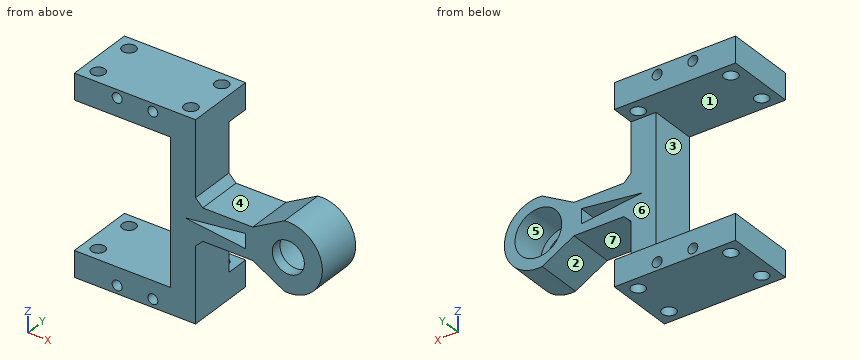
from build123d import *

# Parameters (mm, degrees)
SKETCH8_R                      = 4.5
SKETCH8_R_2                    = 1.4
BOSS_EXTRUDE2_DEPTH            = 19.5
SKETCH10_R                     = 6.55
CUT_EXTRUDE6_DEPTH             = 16.5
CUT_EXTRUDE7_DEPTH             = 43
CUT_EXTRUDE7_DEPTH_BACK        = 47
SKETCH12_R                     = 1.9
CUT_EXTRUDE8_REACH             = 79.29
SKETCH13_W                     = 46.335828735
SKETCH13_H                     = 6.5
CUT_EXTRUDE8_DIRECTION_2_REACH = 79.29
CHAMFER2_SIZE                  = 2
CUT_EXTRUDE9_DEPTH             = 13


with BuildPart() as part:
    # Sketch8 → Boss-Extrude2 (new body)
    with BuildSketch(Plane(origin=(0, 0, 0), x_dir=(1, 0, 0), z_dir=(0, 1, 0))):
        with BuildLine():
            Line((34, 4.5), (50, 4.5))
            Line((50, 4.5), (58.907986832, 9.487360394))
            ThreePointArc((58.907986832, 9.487360394), (69.55, 0), (58.907986832, -9.487360394))
            Line((58.907986832, -9.487360394), (50, -4.5))
            Line((50, -4.5), (34, -4.5))
            Line((34, -4.5), (34, -27.5))
            Line((34, -27.5), (0, -27.5))
            Line((0, -27.5), (0, -20.25))
            Line((0, -20.25), (27, -20.25))
            Line((27, -20.25), (27, 20.25))
            Line((27, 20.25), (0, 20.25))
            Line((0, 20.25), (0, 27.5))
            Line((0, 27.5), (34, 27.5))
            Line((34, 27.5), (34, 4.5))
        make_face()
        with Locations(Location((60, 0, 0), (0, 0, 270))):
            Circle(SKETCH8_R, mode=Mode.SUBTRACT)
        with Locations(Location((22, 25.25, 0), (0, 0, 270))):
            Circle(SKETCH8_R_2, mode=Mode.SUBTRACT)
        with Locations(Location((12, 25.25, 0), (0, 0, 270))):
            Circle(SKETCH8_R_2, mode=Mode.SUBTRACT)
        with Locations(Location((22, -25.25, 0), (0, 0, 270))):
            Circle(SKETCH8_R_2, mode=Mode.SUBTRACT)
        with Locations(Location((12, -25.25, 0), (0, 0, 270))):
            Circle(SKETCH8_R_2, mode=Mode.SUBTRACT)
    extrude(amount=BOSS_EXTRUDE2_DEPTH)

    # Sketch10 → Cut-Extrude6 (cut)
    with BuildSketch(Plane(origin=(0, 19.5, 0), x_dir=(1, 0, 0), z_dir=(0, 1, 0))):
        with Locations(Location((60, 0, 0), (0, 0, 270))):
            Circle(SKETCH10_R)
    extrude(amount=-CUT_EXTRUDE6_DEPTH, mode=Mode.SUBTRACT)

    # Sketch12 → Cut-Extrude7 (cut, two sides: drawn at the far end of the back side and taken through both)
    with BuildSketch(Plane.XY.offset(-CUT_EXTRUDE7_DEPTH_BACK)):
        with Locations(Location((4, 15.75, 0), (0, 0, 180))):
            Circle(SKETCH12_R)
        with Locations(Location((4, 3.75, 0), (0, 0, 180))):
            Circle(SKETCH12_R)
        with Locations(Location((30, 15.75, 0), (0, 0, 180))):
            Circle(SKETCH12_R)
        with Locations(Location((30, 3.75, 0), (0, 0, 180))):
            Circle(SKETCH12_R)
    extrude(amount=CUT_EXTRUDE7_DEPTH + CUT_EXTRUDE7_DEPTH_BACK, mode=Mode.SUBTRACT)

    # Cut-Extrude8: up to this face of the body (flat: up to its plane)
    cut_extrude8_end = Plane(part.part.faces().sort_by_distance((13.927698034, 9.75, -20.25))[0])
    # Sketch13 → Cut-Extrude8 (cut, up to the picked face)
    with BuildSketch(Plane.XY, mode=Mode.PRIVATE) as cut_extrude8_sk1:
        with Locations((46.382085633, 16.25)):
            Rectangle(SKETCH13_W, SKETCH13_H)
    cut_extrude8_tool1 = split(extrude(cut_extrude8_sk1.sketch, amount=-CUT_EXTRUDE8_REACH, mode=Mode.PRIVATE), bisect_by=cut_extrude8_end, keep=Keep.BOTH, mode=Mode.PRIVATE)
    add(cut_extrude8_tool1.solids().sort_by(Axis((46.382086, 16.25, 0), (0, 0, -1)))[0], mode=Mode.SUBTRACT)

    # Cut-Extrude8 direction 2: up to this face of the body (flat: up to its plane)
    cut_extrude8_direction_2_end = Plane(part.part.faces().sort_by_distance((13.927698034, 9.75, 20.25))[0])
    # Sketch13 → Cut-Extrude8 direction 2 (cut, up to the picked face)
    with BuildSketch(Plane.XY, mode=Mode.PRIVATE) as cut_extrude8_direction_2_sk1:
        with Locations((46.382085633, 16.25)):
            Rectangle(SKETCH13_W, SKETCH13_H)
    cut_extrude8_direction_2_tool1 = split(extrude(cut_extrude8_direction_2_sk1.sketch, amount=CUT_EXTRUDE8_DIRECTION_2_REACH, mode=Mode.PRIVATE), bisect_by=cut_extrude8_direction_2_end, keep=Keep.BOTH, mode=Mode.PRIVATE)
    add(cut_extrude8_direction_2_tool1.solids().sort_by(Axis((46.382086, 16.25, 0), (0, 0, 1)))[0], mode=Mode.SUBTRACT)

    # Chamfer2
    chamfer2_edges = [part.edges().sort_by_distance(p)[0] for p in [
        (34, 6.5, 4.5),
        (34, 6.5, -4.5),
    ]]
    chamfer(chamfer2_edges, length=CHAMFER2_SIZE)

    # Sketch16 → Cut-Extrude9 (cut)
    with BuildSketch(Plane(origin=(0, 0, 0), x_dir=(1, 0, 0), z_dir=(0, 1, 0))):
        Polygon((47.953686356, -2.047894041), (47.953686356, 2.047894041), (30.934643554, 0), align=None)
    extrude(amount=CUT_EXTRUDE9_DEPTH, mode=Mode.SUBTRACT)


solid = part.part
The listing builds one solid part. Answer for the finished solid, in the listing's coordinates (mm). Face numbers are marked on the shaded views. A direction names the side the tool comes from. Round coordinates to 2 decimals unless told otherwise and drop trailing zeros. Loops run counter-clockwise (first coordinate to the right, second up) from the corner with the lowest first, then second, coordinate; pieces in that order, holes last. Notation, with made-up numbers: M 19,15 L 47,15 A19 ccw 47,44 Z; hole C -6,36.25 d4. An arc over 180 degrees is marked long. Write each question's results on one line, items separated by ' | '. Start each with the question number.
1) Determine the mould class of the marked faces 1, 2 and 3 for opening direction X: pulls with the +X half, pulls with the -X half, needs draft (parallel to the pull), parting line crosses it, or undercut.
2) Straight lines are drawn through the part: probe 1 along Y at (x, z) = (4, 25.5); probe 2 along X at (y, z) = (11.5, 25.25); probe 3 along Z at (x, y) = (60, 6.75). For each, find the intervals that lie inside material, in ascending order.
3) Find section A-A on z = 25.25. Write down the section's boundary in (x, y), plus the area to 3 significant figures.
4) Find section C-C on x = 30. Write down the section's boundary in (y, z).
5) Which of the six approach directions +Z, -Z, +X, -X, +Y, -Y give full straight-line access (tool end or side, diameter ignored) to the marked faces 4, 5, 6 and 7?
6) Find section B-B on y = 15.75. Count the separate pieces of the cut face and the enclosed holes in it, plus the area to 3 significant figures.
7) Each of these flat-tipped pins is pushed along its axis until it touches: pin 1 (10 mm diameter, centred on y = 5, z = 19.5, fed in from +X); pin 2 (10 mm diameter, centred on x = 47.5, y = 11, fed in from -Z); pin 3 (4 mm diameter, centred on x = 46, y = 6.5, fed in from -Z). Where does it stop, or does it pass through?
8) Find section D-D on y = 10.5. Write down the section's boundary in (x, z).
Final values:
1) face 1: needs draft | face 2: undercut | face 3: pulls with the -X half
2) probe 1: 0 to 1.85, 5.65 to 13.85, 17.65 to 19.5 | probe 2: 0 to 10.6, 13.4 to 20.6, 23.4 to 34 | probe 3: -9.55 to -6.55, 6.55 to 9.55
3) outline: M 0,0 L 10.6,0 L 10.6,19.5 L 0,19.5 Z; M 13.4,0 L 20.6,0 L 20.6,19.5 L 13.4,19.5 Z; M 23.4,0 L 34,0 L 34,19.5 L 23.4,19.5 Z; hole C 4,3.75 d3.8; hole C 4,15.75 d3.8; hole C 30,3.75 d3.8; hole C 30,15.75 d3.8 | area: 508 mm²
4) outline: M 0,-27.5 L 1.85,-27.5 L 1.85,27.5 L 0,27.5 Z; M 5.65,-27.5 L 13.85,-27.5 L 13.85,-20.25 L 13,-20.25 L 13,20.25 L 13.85,20.25 L 13.85,27.5 L 5.65,27.5 Z; M 17.65,-27.5 L 19.5,-27.5 L 19.5,-20.25 L 17.65,-20.25 Z; M 17.65,20.25 L 19.5,20.25 L 19.5,27.5 L 17.65,27.5 Z
5) face 4: +Z, +Y, -Y | face 5: +Y | face 6: +X, -X, +Y | face 7: -Z, +Y, -Y
6) separate pieces: 6 | enclosed holes: 4 | area: 358 mm²
7) pin 1: x = 34 | pin 2: z = -5.9 | pin 3: z = -4.5
8) outline: M 0,-27.5 L 34,-27.5 L 34,-6.5 L 36,-4.5 L 50,-4.5 L 58.91,-9.49 A9.55 ccw long 58.91,9.49 L 50,4.5 L 36,4.5 L 34,6.5 L 34,27.5 L 0,27.5 L 0,20.25 L 27,20.25 L 27,-20.25 L 0,-20.25 Z; hole C 12,-25.25 d2.8; hole C 12,25.25 d2.8; hole C 22,-25.25 d2.8; hole C 22,25.25 d2.8; hole M 30.93,0 L 47.95,-2.05 L 47.95,2.05 Z; hole C 60,0 d13.1
